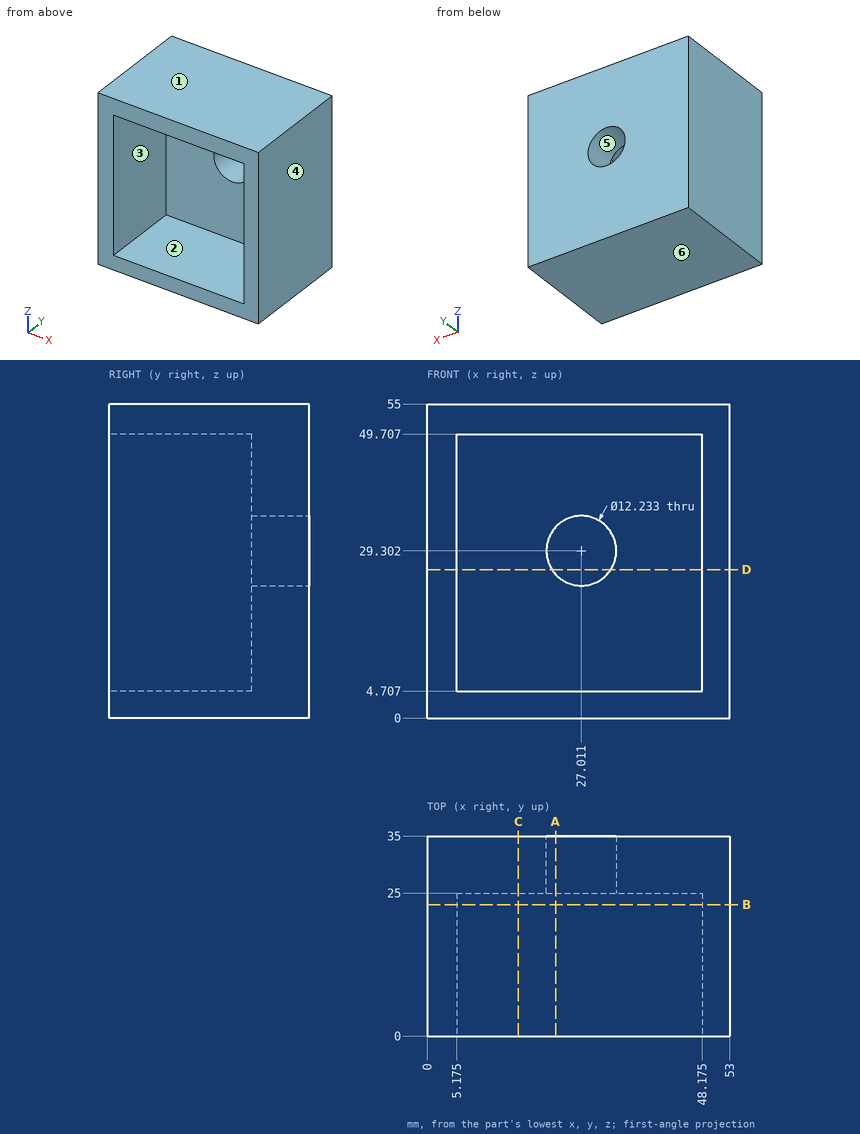
Input: dimensioned drawing with shaded views. Units: mm. Origin: part minimum x, y, z. A direction names the side the tool comes from. Coordinates: 2 decimals unless noted, no trailing zeros. Write each loop counter-clockwise with the first axis right and the second up, starting at its lowest first coordinate (ties: lowest second). Pieces come first, ordered by that corner, then holes. Notation, with made-up numbers: M 88,17.5 L 147,17.5 A19 cw 147,24.5 Z; hole C -9.75,45 d9. An arc over 180 degrees is marked long. Answer as a JSON object with one key per item and string values. Group by question number.
(1) Ray query, line 1 along X through (y, z) = (6, 11.5) (1 decimal); line 2 along Z through (x, y) = (16.5, 3.5); line 3 along Y through (x, z) = (33.5, 7). Return the intervals inside material, ascending. Write a range as [from, to].
(2) Section D-D on z = 26. Output: boundary loops of the cut face in (x, y) (1 decimal), plus the area to 3 significant figures.
(3) Section B-B on y = 23. Output: boundary loops of the cut face in (x, z) (1 decimal), plus the area to 3 significant figures.
(4) Mould query, pull axis X, two halves, no side actions, for the marked faces 3, 4, 5 and 6. Classes: pulls with the +X half, pulls with the -X half, needs draft (parallel to the pull), parting line crosses it, or undercut.
(5) Set-up query: the marked faces 1 and 2. Return all of +Z, -Z, +X, -X, +Y, -Y with unobstructed straight access to the full face (end or side cutting, diameter ignored); none if empty.
(6) Contact query for a flat-ended pin moving along its axis: P1, Ø2, axis at x = 47, z = 26, coming from the -Y side. Output: stop coordinate, or through.
(7) Section A-A on x = 22.5. Output: boundary loops of the cut face in (y, z), plus the area to 3 significant figures.
(8) Section C-C on x = 16. Output: boundary loops of the cut face in (y, z), plus the area to 3 significant figures.
Result set:
{
 "1": {"line 1": "x = [0, 5.2], [48.2, 53]", "line 2": "z = [0, 4.71], [49.71, 55]", "line 3": "y = [25, 35]"},
 "2": {"outline": "M 0,0 L 5.2,0 L 5.2,25 L 21.9,25 L 21.9,35 L 0,35 Z; M 32.2,25 L 48.2,25 L 48.2,0 L 53,0 L 53,35 L 32.2,35 Z", "area": "677 mm2"},
 "3": {"outline": "M 0,0 L 53,0 L 53,55 L 0,55 Z; hole M 5.2,4.7 L 48.2,4.7 L 48.2,49.7 L 5.2,49.7 Z", "area": "980 mm2"},
 "4": {"face 3": "undercut", "face 4": "pulls with the +X half", "face 5": "undercut", "face 6": "needs draft"},
 "5": {"face 1": "+Z, +X, -X, +Y, -Y", "face 2": "-Y"},
 "6": {"P1": "stops at y = 25"},
 "7": {"outline": "M 0,0 L 35,0 L 35,25.17 L 25,25.17 L 25,4.71 L 0,4.71 Z; M 0,49.71 L 25,49.71 L 25,33.43 L 35,33.43 L 35,55 L 0,55 Z", "area": "717 mm2"},
 "8": {"outline": "M 0,0 L 35,0 L 35,55 L 0,55 L 0,49.71 L 25,49.71 L 25,4.71 L 0,4.71 Z", "area": "800 mm2"}
}
